Source: CAD feature listing. Evaluate the final solid. Frame: model axes, mm. A direction names the side the tool comes from. Round coordinates to 2 decimals unless told otherwise and drop trailing zeros. Loops run counter-clockwise (first coordinate to the right, second up) from the corner with the lowest first, then second, coordinate; pieces in that order, holes last.
Item 1: Access query for faces 1 (the flat face through (3, -10, -6.5)), 2 (the flat face through (-125, -10, 0)), 3 (the flat face through (-80.5, -10, 12)). Directions: +Z, -Z, +X, -X, +Y, -Y. A direction counts if a zero-diameter tool reaches every point of the face in a straight line with its end or side. Return the directions, or none.
Item 2: Ray query, L1, parallel to X at y = -10.75, z = 0.5; L2, parallel to X at y = -10.25, z = 10; L3, parallel to Y at x = -118, z = -2. Return the intervals inside material, ascending.
Item 3: First-contact query: P1, Ø3.5, axis at x = 2.5, y = -13.5, coming from the +Z side; P2, Ø1.5, axis at x = 3.5, y = -14.5, coming from the -Z side. Flat tips, straight axial feed; report the tip coordinate or a pass-through.
Item 4: Section query B-B on z = -12. Give the number of separate pieces and of enclosed holes in the cut face, then the cut area to 3 significant figures.
Item 5: Section query A-A on z = 12. Return loops of the section in (x, y), then the cut area to 3 significant figures.
Item 6: Section query C-C on x = 3. Return loops of the section in (y, z).
Item 7: Pull-direction query (X, two-part tool) for faces 4 (the flat face through (-38, -10, -16.5)), 5 (the flat face through (0, -10, 6.5)), 6 (the flat face through (78, -10, -6.5)), 7 (the cylindrical face through (123, -19, 0)); classes: released by +X, released by -X, zero draft, split by the parting line, or undercut.
```python
from build123d import *

# Parameters (mm, degrees)
F0_W      = 250
F0_H      = 33
F1_DEPTH  = 20
F2_W      = 11
F2_H      = 20
F4_DEPTH  = 10
F3_W      = 5
F3_H      = 20
F5_DEPTH  = 10
F6_R      = 5
F7_R      = 5
F8_R      = 5
F9_R      = 5
F10_R     = 6
F11_DEPTH = 33.001


with BuildPart() as f1:
    # F0 (on Front) → F1 (new body)
    with BuildSketch(Plane.XZ):
        Rectangle(F0_W, F0_H)
    extrude(amount=F1_DEPTH)

    # F2 (on face) → F4 (cut)
    with BuildSketch(Plane.XY.offset(16.5)):
        with Locations((-75, -10)):
            Rectangle(F2_W, F2_H)
        with Locations((0, -10)):
            Rectangle(F2_W, F2_H)
        with Locations((75, -10)):
            Rectangle(F2_W, F2_H)
    extrude(amount=-F4_DEPTH, mode=Mode.SUBTRACT)

    # F3 (on face) → F5 (cut)
    with BuildSketch(Plane(origin=(0, 0, -16.5), x_dir=(1, 0, 0), z_dir=(0, 0, -1))):
        with Locations((-78.25, 10)):
            Rectangle(F3_W, F3_H)
        with Locations((-71.75, 10)):
            Rectangle(F3_W, F3_H)
        with Locations((-3.25, 10)):
            Rectangle(F3_W, F3_H)
        with Locations((3.25, 10)):
            Rectangle(F3_W, F3_H)
        with Locations((71.75, 10)):
            Rectangle(F3_W, F3_H)
        with Locations((78.25, 10)):
            Rectangle(F3_W, F3_H)
    extrude(amount=-F5_DEPTH, mode=Mode.SUBTRACT)

    # F6
    f6_edges = [f1.edges().sort_by_distance(p)[0] for p in [
        (-125, -20, 0),
    ]]
    fillet(f6_edges, radius=F6_R)

    # F7
    f7_edges = [f1.edges().sort_by_distance(p)[0] for p in [
        (-125, 0, 0),
    ]]
    fillet(f7_edges, radius=F7_R)

    # F8
    f8_edges = [f1.edges().sort_by_distance(p)[0] for p in [
        (125, -20, 0),
    ]]
    fillet(f8_edges, radius=F8_R)

    # F9
    f9_edges = [f1.edges().sort_by_distance(p)[0] for p in [
        (125, 0, 0),
    ]]
    fillet(f9_edges, radius=F9_R)

    # F10 (on face) → F11 (cut, through all)
    with BuildSketch(Plane.XY.offset(16.5)):
        with Locations((118, -10)):
            Circle(F10_R)
        with Locations((-118, -10)):
            Circle(F10_R)
    extrude(amount=-F11_DEPTH, mode=Mode.SUBTRACT)


solid = f1.part
```
Data:
1. face 1: -Z, +Y, -Y
1. face 2: +Z, -Z, -X, +Y, -Y
1. face 3: +Z, +Y, -Y
2. L1: x = -125 to -123.95, -112.05 to 112.05, 123.95 to 125
2. L2: x = -125 to -123.99, -112.01 to -80.5, -69.5 to -5.5, 5.5 to 69.5, 80.5 to 112.01, 123.99 to 125
2. L3: y = -20 to -16, -4 to 0
3. P1: stops at z = 6.5
3. P2: stops at z = -6.5
4. separate pieces: 7
4. enclosed holes: 2
4. area: 4,150 mm2
5. outline: (-125, -15) arc R5 ccw to (-120, -20) - (-80.5, -20) - (-80.5, 0) - (-120, 0) arc R5 ccw to (-125, -5) - close; (-69.5, -20) - (-5.5, -20) - (-5.5, 0) - (-69.5, 0) - close; (5.5, -20) - (69.5, -20) - (69.5, 0) - (5.5, 0) - close; (80.5, -20) - (120, -20) arc R5 ccw to (125, -15) - (125, -5) arc R5 ccw to (120, 0) - (80.5, 0) - close; hole circle Ø12 at (-118, -10); hole circle Ø12 at (118, -10)
5. area: 4,090 mm2
6. outline: (-20, -6.5) - (0, -6.5) - (0, 6.5) - (-20, 6.5) - close
7. face 4: zero draft
7. face 5: undercut
7. face 6: undercut
7. face 7: released by +X
